Geometry: final body of the model. Coordinates: model frame, mm. Face numbers are marked on the shaded views. A direction names the side the tool comes from. Give positions to 0.01 mm unless a question says otherwise; leave off trailing zeros. Loops run counter-clockwise (first coordinate to the right, second up) from the corner with the lowest first, then second, coordinate; pieces in that order, holes last.
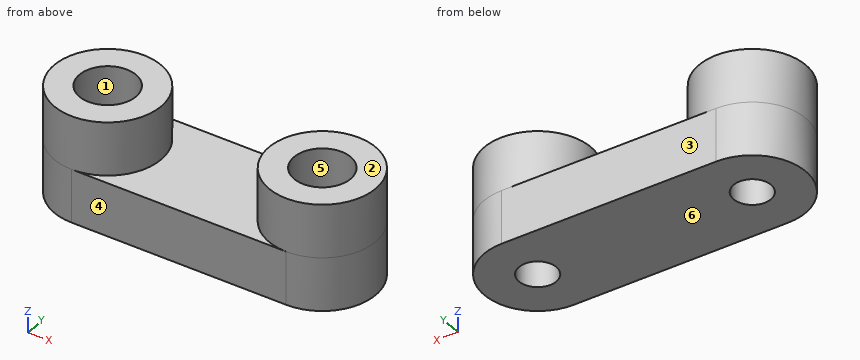
```python
from build123d import *

# Parameters (mm, degrees)
ESTRUSIONE_ESTRUSIONE1_DEPTH = 5
SCHIZZO2_R                   = 5
SCHIZZO2_R_2                 = 2.65
ESTRUSIONE_ESTRUSIONE2_DEPTH = 5
SCHIZZO3_R                   = 1.75
TAGLIO_ESTRUSIONE1_DEPTH     = 6


with BuildPart() as part:
    # Schizzo1 → Estrusione-Estrusione1 (new body)
    with BuildSketch(Plane.XY):
        with BuildLine():
            Line((-7.862204724, 5), (12.137795276, 5))
            ThreePointArc((12.137795276, 5), (17.137795276, 0), (12.137795276, -5))
            Line((12.137795276, -5), (-7.862204724, -5))
            ThreePointArc((-7.862204724, -5), (-12.862204724, 0), (-7.862204724, 5))
        make_face()
    extrude(amount=ESTRUSIONE_ESTRUSIONE1_DEPTH)

    # Schizzo2 → Estrusione-Estrusione2 (add)
    with BuildSketch(Plane.XY.offset(5)):
        with Locations((-7.862204724, 0)):
            Circle(SCHIZZO2_R)
        with Locations((-7.862204724, 0)):
            Circle(SCHIZZO2_R_2, mode=Mode.SUBTRACT)
        with Locations((12.137795276, 0)):
            Circle(SCHIZZO2_R)
        with Locations((12.137795276, 0)):
            Circle(SCHIZZO2_R_2, mode=Mode.SUBTRACT)
    extrude(amount=ESTRUSIONE_ESTRUSIONE2_DEPTH)

    # Schizzo3 → Taglio-Estrusione1 (cut, through all)
    with BuildSketch(Plane.XY.offset(5)):
        with Locations((-7.862204724, 0)):
            Circle(SCHIZZO3_R)
        with Locations((12.137795276, 0)):
            Circle(SCHIZZO3_R)
    extrude(amount=-TAGLIO_ESTRUSIONE1_DEPTH, mode=Mode.SUBTRACT)


solid = part.part
```
Q1. Section query C-C, the plane x = -1.5. Return loops of the section in (y, z), and give its area (3 significant figures).
Q2. Section query D-D, the plane y = 3. Return loops of the section in (x, z), and give its area (3 significant figures).
Q3. Pin query (flat end, axial travel): pin 1 Ø1.5 at (y, z) = (-2.5, 1.5) entering from +X; pin 2 Ø2 at (x, y) = (12.14, 0) entering from -Z; pin 3 Ø4 at (x, y) = (12, 0) entering from +Z; pin 4 Ø1.5 at (y, z) = (3, 8) entering from +X. Return the tip coordinate at first contact, or that it passes through.
Q4. Reachability of the marked faces 5 and 6 from +Z, -Z, +X, -X, +Y, -Y: full face, straight path, thin tool, end or side. Return the list, or none.
Q5. Material intervals for probe 1 along X at (y, z) = (-1.5, 7); probe 2 along Z at (x, y) = (8.25, 4); probe 3 along X at (y, z) = (-1, 0.75), sorted ascending.
Q6. Section query A-A, the plane y = 0. Return loops of the section in (x, z).
Q7. Section query B-B, the plane z = 7.5. Return loops of the section in (x, y), and give its area (3 significant figures).
Q8. Mould query, pull axis Y, two halves, no side actions, for the marked faces 1, 2, 3 and 4. Classes: +Y half, -Y half, draft (parallel to the pull), parting line (faces both ways), or undercut.
Resolved:
1. outline: (-5, 0) - (5, 0) - (5, 5) - (-5, 5) - close
1. area: 50.0 mm2
2. outline: (-11.86, 0) - (16.14, 0) - (16.14, 10) - (8.14, 10) - (8.14, 5) - (-3.86, 5) - (-3.86, 10) - (-11.86, 10) - close
2. area: 220 mm2
3. pin 1: stops at x = 16.82
3. pin 2: passes through
3. pin 3: stops at z = 5
3. pin 4: stops at x = 16.6
4. face 5: +Z
4. face 6: -Z, +X, -X, +Y, -Y
5. probe 1: x = -12.63 to -10.05, -5.68 to -3.09, 7.37 to 9.95, 14.32 to 16.91
5. probe 2: z = 0 to 5
5. probe 3: x = -12.76 to -9.3, -6.43 to 10.7, 13.57 to 17.04
6. outline: (-12.86, 0) - (-9.61, 0) - (-9.61, 5) - (-10.51, 5) - (-10.51, 10) - (-12.86, 10) - close; (-6.11, 0) - (10.39, 0) - (10.39, 5) - (9.49, 5) - (9.49, 10) - (7.14, 10) - (7.14, 5) - (-2.86, 5) - (-2.86, 10) - (-5.21, 10) - (-5.21, 5) - (-6.11, 5) - close; (13.89, 0) - (17.14, 0) - (17.14, 10) - (14.79, 10) - (14.79, 5) - (13.89, 5) - close
7. outline: circle Ø10 at (-7.86, 0); circle Ø10 at (12.14, 0); hole circle Ø5.3 at (-7.86, 0); hole circle Ø5.3 at (12.14, 0)
7. area: 113 mm2
8. face 1: undercut
8. face 2: draft
8. face 3: +Y half
8. face 4: -Y half
